```python
from build123d import *

# Parameters (mm, degrees)
SKETCH1_W               = 171
SKETCH1_H               = 61
SKETCH1_W_2             = 165
SKETCH1_H_2             = 55
BOSS_EXTRUDE1_DEPTH     = 10
SKETCH2_W               = 200
SKETCH2_H               = 100
BOSS_EXTRUDE2_DEPTH     = 5
FILLET1_R               = 1
F_10_0MM_DOWEL_HOLE1_D  = 10
FILLET2_R               = 1
CUT_EXTRUDE2_DEPTH      = 113.249721603
CUT_EXTRUDE2_DEPTH_BACK = 113.249721603
SKETCH5_W               = 155
SKETCH5_H               = 45


with BuildPart() as part:
    # Sketch1 → Boss-Extrude1 (new body)
    with BuildSketch(Plane(origin=(0, 0, 0), x_dir=(1, 0, 0), z_dir=(0, 1, 0))):
        Rectangle(SKETCH1_W, SKETCH1_H)
        Rectangle(SKETCH1_W_2, SKETCH1_H_2, mode=Mode.SUBTRACT)
    extrude(amount=BOSS_EXTRUDE1_DEPTH)

    # Sketch2 → Boss-Extrude2 (add)
    with BuildSketch(Plane(origin=(0, 0, 0), x_dir=(1, 0, 0), z_dir=(0, 1, 0))):
        Rectangle(SKETCH2_W, SKETCH2_H)
    extrude(amount=-BOSS_EXTRUDE2_DEPTH)

    # Fillet1
    fillet1_edges = [part.edges().sort_by_distance(p)[0] for p in [
        (0, 10, 30.5),
        (82.5, 10, 0),
        (85.5, 10, 0),
        (0, 10, -27.5),
        (-82.5, 10, 0),
        (0, 10, 27.5),
        (0, 10, -30.5),
        (-85.5, 10, 0),
    ]]
    fillet(fillet1_edges, radius=FILLET1_R)

    # Ø10.0mm Dowel Hole1 (through all)
    with Locations(Plane(origin=(-87.5, 0, -37.5), x_dir=(0, 0, 1), z_dir=(0, 1, 0))):
        with Locations((0, 0), (0, 175), (75, 175), (75, 0)):
            Hole(F_10_0MM_DOWEL_HOLE1_D / 2)

    # Fillet2
    fillet2_edges = [part.edges().sort_by_distance(p)[0] for p in [
        (100, 0, 0),
        (0, 0, -50),
        (-100, 0, 0),
        (0, 0, 50),
        (85.5, 0, 0),
        (0, 0, 30.5),
        (-85.5, 0, 0),
        (0, 0, -30.5),
        (-87.5, 0, 42.5),
        (87.5, 0, 42.5),
        (87.5, 0, -32.5),
        (-87.5, 0, -32.5),
    ]]
    fillet(fillet2_edges, radius=FILLET2_R)

    # Sketch5 → Cut-Extrude2 (cut, two sides: drawn at the far end of the back side and taken through both)
    with BuildSketch(Plane(origin=(0, 0, 0), x_dir=(1, 0, 0), z_dir=(0, 1, 0)).offset(-CUT_EXTRUDE2_DEPTH_BACK)):
        Rectangle(SKETCH5_W, SKETCH5_H)
    extrude(amount=CUT_EXTRUDE2_DEPTH + CUT_EXTRUDE2_DEPTH_BACK, mode=Mode.SUBTRACT)


solid = part.part
```
Geometry check sheet. Reference: the model listing, model coordinates, mm. A direction names the side the tool comes from. Round coordinates to 2 decimals unless told otherwise and drop trailing zeros. Loops run counter-clockwise (first coordinate to the right, second up) from the corner with the lowest first, then second, coordinate; pieces in that order, holes last. Notation, with made-up numbers: (-19.5, -30.75) -> (6.5, -30.75) arc R25 ccw to (6.5, -0.75) -> close; hole circle Ø3 at (35, 32). An arc over 180 degrees is marked (long way). Use a Markdown table: item, result.
(1) Sectioned sample at A-A (z = 20). Enter the section's corners in (x, y), then the cut area to 3 significant figures.
Calculated:
| item | result |
|---|---|
| outline | (-100, -5) -> (-77.5, -5) -> (-77.5, 0) -> (-82.5, 0) -> (-82.5, 9) arc R1 ccw to (-83.5, 10) -> (-84.5, 10) arc R1 ccw to (-85.5, 9) -> (-85.5, 1) arc R1 cw to (-86.5, 0) -> (-99, 0) arc R1 ccw to (-100, -1) -> close; (77.5, -5) -> (100, -5) -> (100, -1) arc R1 ccw to (99, 0) -> (86.5, 0) arc R1 cw to (85.5, 1) -> (85.5, 9) arc R1 ccw to (84.5, 10) -> (83.5, 10) arc R1 ccw to (82.5, 9) -> (82.5, 0) -> (77.5, 0) -> close |
| area | 284 mm² |
(2) Sectioned sample at C-C (z = -37.5). Enter the section's corners in (x, y).
Calculated:
| item | result |
|---|---|
| outline | (-100, -5) -> (-92.5, -5) -> (-92.5, -1) arc R1 ccw to (-93.5, 0) -> (-99, 0) arc R1 ccw to (-100, -1) -> close; (-82.5, -5) -> (82.5, -5) -> (82.5, -1) arc R1 ccw to (81.5, 0) -> (-81.5, 0) arc R1 ccw to (-82.5, -1) -> close; (92.5, -5) -> (100, -5) -> (100, -1) arc R1 ccw to (99, 0) -> (93.5, 0) arc R1 ccw to (92.5, -1) -> close |
(3) Scan lines: probe 1 along X at (y, z) = (-2.85, 37.5); probe 2 along Z at (x, y) = (6.5, 2.75); probe 3 along X at (y, z) = (-1.5, 6). Record each from-to range of solid material in increasing order.
Calculated:
| item | result |
|---|---|
| probe 1 | -100 to -92.5, -82.5 to 82.5, 92.5 to 100 |
| probe 2 | -30.5 to -27.5, 27.5 to 30.5 |
| probe 3 | -100 to -77.5, 77.5 to 100 |
(4) Sectioned sample at B-B (x = 2.5). Enter the section's corners in (y, z).
Calculated:
| item | result |
|---|---|
| outline | (-5, -50) -> (-1, -50) arc R1 ccw to (0, -49) -> (0, -31.5) arc R1 cw to (1, -30.5) -> (9, -30.5) arc R1 ccw to (10, -29.5) -> (10, -28.5) arc R1 ccw to (9, -27.5) -> (0, -27.5) -> (0, -22.5) -> (-5, -22.5) -> close; (-5, 22.5) -> (0, 22.5) -> (0, 27.5) -> (9, 27.5) arc R1 ccw to (10, 28.5) -> (10, 29.5) arc R1 ccw to (9, 30.5) -> (1, 30.5) arc R1 cw to (0, 31.5) -> (0, 49) arc R1 ccw to (-1, 50) -> (-5, 50) -> close |
(5) Set-up check for faces 4 (the flat face through (77.5, -3, 0)), 5 (the flat face through (-85.5, 5, 0)), 6 (the flat face through (-1, 4, -27.5)): record each of +Z, -Z, +X, -X, +Y, -Y from which the full face is reachable in a straight line by a thin tool's end or side.
Calculated:
| item | result |
|---|---|
| face 4 | +Y, -Y |
| face 5 | +Z, -Z, -X, +Y |
| face 6 | +Y |
(6) Sectioned sample at D-D (y = 3.5). Enter the section's corners in (x, z), then the cut area to 3 significant figures.
Calculated:
| item | result |
|---|---|
| outline | (-85.5, -30.5) -> (85.5, -30.5) -> (85.5, 30.5) -> (-85.5, 30.5) -> close; hole (-82.5, -27.5) -> (82.5, -27.5) -> (82.5, 27.5) -> (-82.5, 27.5) -> close |
| area | 1,360 mm² |
(7) Go/stop test with flat-tipped pins: P1, Ø4, axis at y = 4.5, z = 10, coming from the +X side; P2, Ø6.5, axis at x = 0.5, y = 5, coming from the +Z side; P3, Ø1.5, axis at y = 4.5, z = -26.5, coming from the -X side. Record where each tip stops, or that it passes through.
Calculated:
| item | result |
|---|---|
| P1 | x = 85.5 |
| P2 | z = 30.5 |
| P3 | x = -85.5 |
(8) Mould release check, pull along X, two halves, no side actions. Record for faces 1 (the flat face through (85.5, 5, 0)), 2 (the flat face through (0, 10, -29)), 3 (the flat face through (-1, -3, -22.5)): released by +X, released by -X, zero draft, split by the parting line, or undercut.
Calculated:
| item | result |
|---|---|
| face 1 | released by +X |
| face 2 | zero draft |
| face 3 | undercut |
